Autodesk Inventor part; units mm, degrees
ref_plane "Work Plane1" through (3, 0, 0) normal (0, 0.5, 0.866) x (1, 0, 0)
ref_plane "YZ Plane" through (0, 0, 0) normal (1, 0, 0) x (0, 1, 0)
ref_plane "XZ Plane" through (0, 0, 0) normal (0, 1, 0) x (-1, 0, 0)
sketch "Sketch1" plane through (0, 0, 0) normal (0, 0, 1) x (1, 0, 0)
  line L0 (0, 4) -> (0, 0)
  line L1 (0, 0) -> (20, 0)
  line L2 (20, 0) -> (20, 4)
  line L3 (20, 4) -> (0, 4)
  line L4 (-4, 0) -> (24, 0)
  line L5 (0, -0.8) -> (0, 4.8)
  dimension "d0" = 8
  dimension "d1" = 20
revolve "Body" add sketch "Sketch1" angle 360 about axis through (0, 0, 0) along (1, 0, 0)
sketch "Sketch2" plane through (0, 0, 0) normal (1, 0, 0) x (0, 1, 0)
  line L0 (0, 7.5056) -> (6.5, 3.7528)
  line L1 (6.5, 3.7528) -> (6.5, -3.7528)
  line L2 (6.5, -3.7528) -> (0, -7.5056)
  line L3 (0, -7.5056) -> (-6.5, -3.7528)
  line L4 (-6.5, -3.7528) -> (-6.5, 3.7528)
  line L5 (-6.5, 3.7528) -> (0, 7.5056)
  line L6 (-9.1, 0) -> (9.1, 0)
  line L7 (0, -10.5078) -> (0, 10.5078)
  point P0 (0, 0)
  point P1 (0, 0)
  dimension "d2" = 13
extrude "Head" add sketch "Sketch2" against normal blind 6.5
sketch "Sketch3" plane through (-6.5, 0, 0) normal (-1, 0, 0) x (0, 1, 0)
  circle A0 centre (0, 0) radius 4.875
  point P0 (0, 0)
  dimension "d12" = 9.75
extrude "Indent1" cut sketch "Sketch3" against normal blind 1.3
sketch "Sketch4" plane through (0, 0, 0) normal (0, 0, 1) x (1, 0, 0)
  line L0 (-6.5, 7.5056) -> (-6.5, 6.5)
  line L1 (-6.5, 6.5) -> (-5.9194, 7.5056)
  line L2 (-5.9194, 7.5056) -> (-6.5, 7.5056)
  line L3 (0, 7.5056) -> (0, 6.5)
  line L4 (0, 6.5) -> (-0.5806, 7.5056)
  line L5 (-0.5806, 7.5056) -> (0, 7.5056)
  line L6 (0, 0) -> (-6.5, 0)
  line L7 (-6.5, 0) -> (-6.5, 6.5)
  line L8 (0, 0) -> (0, 6.5)
  line L9 (-7.8, 0) -> (1.3, 0)
  line L10 (-5.9194, 7.5056) -> (-0.5806, 7.5056) construction
  line L11 (0, -1.5011) -> (0, 9.0067)
  dimension "d6" = 30
  dimension "d7" = 30
  dimension "d16" = 13
  dimension "d17" = 13
  dimension "d18" = 15.0111
revolve "Chamfer1" cut sketch "Sketch4" angle 360 about axis through (-10, 0, 0) along (1, 0, 0)
fillet "Fillet1" radius 0.4 1 edges at (0, -4, 0)
thread "Thread"
ref_plane "Work Plane1" through (3, 0, 0) normal (0, 0.5, 0.866) x (1, 0, 0)
equation "\"d0\" = GD"
equation "\"d1\" = NLG"
equation "\"d2\" = SW"
equation "\"d3\" = KOH"
equation "\"d12\" = 0.75 * SW0"
equation "\"d14\" = 0.2 * KOH"
equation "\"d6\" = ANG1"
equation "\"d7\" = ANG1"
equation "\"d16\" = SW0"
equation "\"d17\" = SW0"
equation "\"d18\" = 1.1547 * SW"
equation "\"d11\" = RR"
equation "\"d8\" = GEL"
equation "\"NLG\" = 20"
equation "\"KOH\" = 6.5"
equation "\"GD\" = NND"
equation "\"GEL\" = 17.5"
equation "\"SW\" = 13"
equation "\"SW0\" = SW"
equation "\"ANG1\" = 30deg"
equation "\"RR\" = 0.4"
equation "\"GUL\" = 0.61345 * PTC"
equation "\"SPD\" = NND - 1.2269 * PTC"
equation "\"GD1\" = THREADDIA - 1.2269 * PTC"
equation "\"THREADDIA\" = 8"
equation "\"SDH\" = 9.2"
equation "\"TOA\" = 30deg"
equation "\"BDM\" = NND"
equation "\"FAWI\" = 45deg"
equation "\"PTC\" = 1.25"
equation "\"NND\" = 8"
equation "\"GAL\" = 0.61345 * PTC"
equation "\"SD\" = 0"
equation "\"SD2\" = SDH"
equation "\"E0\" = 1.155 * SW"
properties part number "AS 1427 - M8 x 20" material "Steel, Mild"
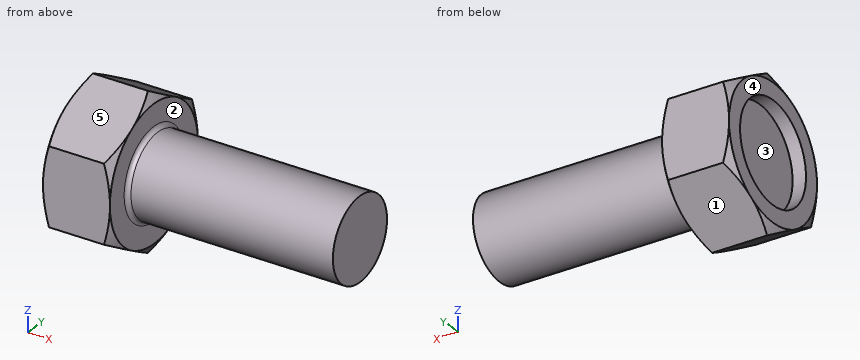
Verification items for the finished model (mm, model axes). Face numbers are marked on the shaded views. A direction names the side the tool comes from. Round coordinates to 2 decimals unless told otherwise and drop trailing zeros. Order: outer loops, then holes, each group sorted by start corner. A loop starts at its lowest first (then second) coordinate and runs counter-clockwise, first axis right, second up.
1) Draft check along Z on the marked faces 3, 4 and 5. Enter one of: +Z half, -Z half, draft (parallel to the pull), parting line (faces both ways), or undercut.
Geometry says:
face 3: undercut
face 4: draft
face 5: +Z half
2) Cross-section at B-B, the plane x = 4.25. Record the cut outline in (y, z), plus the area to 3 significant figures.
Geometry says:
outline: circle Ø8 at (0, 0)
area: 50.3 mm2
3) Tool access check on the marked faces 1 and 2. Record the directions out of +Z, -Z, +X, -X, +Y, -Y that give a thin tool (end or side, any length) a straight path to the whole face; none if there is none.
Geometry says:
face 1: -Z, +X, -X, +Y
face 2: +X
4) Material ranges on line 1 (Y direction, x = -5.9, z = 0) (3 decimals); line 2 (X direction, y = -3.75, z = -0.5); line 3 (X direction, y = 2, z = 5.5), recorded low to high.
Geometry says:
line 1: y = -6.5 to -4.875, 4.875 to 6.5
line 2: x = -5.2 to 20
line 3: x = -6.5 to 0
5) Depth check by flat-ended pin: pin 1 (3 mm diameter, centred on y = -1.5, z = 1, fed in from -X); pin 2 (4 mm diameter, centred on x = 3, z = -3, fed in from +Y); pin 3 (3 mm diameter, centred on x = -2.5, y = 2, fed in from +Z). Enter the tip coordinate at first touch or a pass-through.
Geometry says:
pin 1: stops at x = -5.2
pin 2: stops at y = 3.87
pin 3: stops at z = 7.22
6) Cross-section at A-A, the plane x = -3.25. Record the cut outline in (y, z), plus the area to 3 significant figures.
Geometry says:
outline: (-6.5, -3.75) - (0, -7.51) - (6.5, -3.75) - (6.5, 3.75) - (0, 7.51) - (-6.5, 3.75) - close
area: 146 mm2
